Geometry check sheet. Reference: the model listing, model coordinates, mm. Face numbers are marked on the shaded views. Give positions to 0.01 mm unless a question says otherwise; leave off trailing zeros. Write each loop counter-clockwise with the first axis right and the second up, starting at its lowest first coordinate (ties: lowest second). Pieces come first, ordered by that corner, then holes. Notation, with made-up numbers: (-30.75, 85) -> (-17.75, 85) arc R28 ccw to (-17.75, 119) -> close; hole circle Ø9 at (7.25, 69). An arc over 180 degrees is marked (long way). One line per item, written item: value.
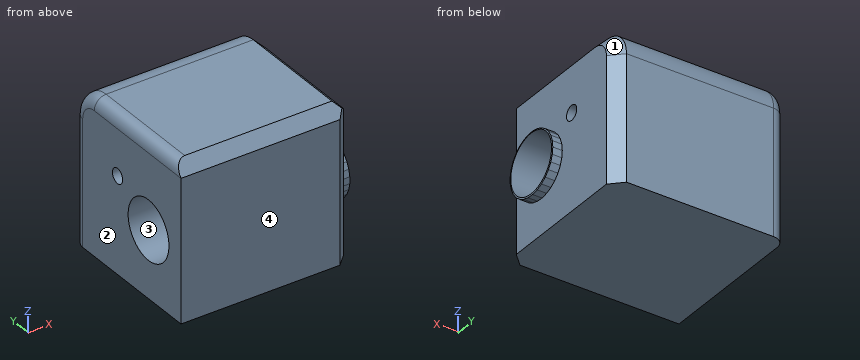
from build123d import *

# Parameters (mm, degrees)
F0_W      = 73.2621699572
F0_H      = 66.2733446807
F1_DEPTH  = 66.04
F2_R      = 12.2642048969
F4_D      = 6.35
F5_SIZE   = 5.08
F6_SIZE   = 5.08
F7_SIZE   = 5.08
F8_R      = 5.08
F10_DEPTH = 4.064
F12_D     = 25.4


with BuildPart() as f1:
    # F0 (on Top) → F1 (new body)
    with BuildSketch(Plane.XY):
        with Locations((2.2894442081, 5.3018676117)):
            Rectangle(F0_W, F0_H)
    extrude(amount=F1_DEPTH)

    # F2
    f2_edges = [f1.edges().sort_by_distance(p)[0] for p in [
        (2.289444, 38.43854, 66.04),
    ]]
    fillet(f2_edges, radius=F2_R)

    # F4 (through all)
    with Locations(Plane(origin=(-34.3416407704, 0, 0), x_dir=(0, -1, 0), z_dir=(-1, 0, 0))):
        with Locations((-11.6805844009, 41.2179939449)):
            Hole(F4_D / 2)

    # F5
    f5_edges = [f1.edges().sort_by_distance(p)[0] for p in [
        (2.289444, -27.834805, 66.04),
    ]]
    chamfer(f5_edges, length=F5_SIZE)

    # F6
    f6_edges = [f1.edges().sort_by_distance(p)[0] for p in [
        (38.920529, -27.834805, 30.48),
    ]]
    chamfer(f6_edges, length=F6_SIZE)

    # F7
    f7_edges = [f1.edges().sort_by_distance(p)[0] for p in [
        (38.920529, 34.846438, 62.447898),
    ]]
    chamfer(f7_edges, length=F7_SIZE)

    # F8
    f8_edges = [f1.edges().sort_by_distance(p)[0] for p in [
        (-34.341641, 34.846438, 62.447898),
    ]]
    fillet(f8_edges, radius=F8_R)

    # F9 (on face) → F10 (join)
    with BuildSketch(Plane.YZ.offset(38.9205291867)):
        Polygon((-1.1907316289, 16.7186320739), (1.1907316289, 18.3312571628), (3.169850874, 20.4181241781), (4.6540846899, 22.8816535376), (5.5740319532, 25.6066533465), (5.8866769522, 28.4657056424), (5.5774007542, 31.3251243174), (4.6606647705, 34.0512061324), (3.1793345569, 36.5164825315), (1.2026754677, 38.6056799302), (-1.1768861149, 40.2211097802), (-3.848084536, 41.2872363771), (-6.6860175264, 41.7542088262), (-9.5579864934, 41.6001920146), (-12.3297013601, 40.8323875974), (-14.87155982, 39.4866972558), (-17.0647073965, 37.6260439744), (-18.8065949465, 35.3374298329), (-20.015773744, 32.7278678847), (-20.6357039325, 29.9193783463), (-20.6373982652, 27.0432830671), (-20.0207775172, 24.2340650658), (-18.8146741891, 21.623080254), (-17.0754843323, 19.3324153794), (-14.8845305313, 17.4691793858), (-12.3442593509, 16.1204951174), (-9.5734510482, 15.3494255516), (-6.7016655399, 15.1920250443), (-3.8631843245, 15.6556534684), align=None)
    extrude(amount=F10_DEPTH)

    # F12 (through all)
    with Locations(Plane.YZ.offset(42.9845291867)):
        with Locations((-7.5925402343, 28.6855231971)):
            Hole(F12_D / 2)


solid = f1.part
1) Depth check by flat-ended pin: pin 1 Ø1 at (x, y) = (30, -2) entering from -Z; pin 2 Ø8 at (y, z) = (-7, 10.5) entering from +X. Enter the tip coordinate at first touch or a pass-through.
Verdict:
pin 1: z = 0
pin 2: x = 38.92
2) Sectioned sample at A-A on x = 32. Record the cut outline in (y, z) (3 decimals).
Verdict:
outline: (-27.835, 0) -> (38.439, 0) -> (38.439, 53.776) arc R12.264 ccw to (26.174, 66.04) -> (-22.755, 66.04) -> (-27.835, 60.96) -> close; hole circle Ø25.4 at (-7.593, 28.686); hole circle Ø6.35 at (11.681, 41.218)
3) Mould release check, pull along Y, two halves, no side actions. Record for the marked faces 1, 2, 3 and 4: released by +Y, released by -Y, zero draft, split by the parting line, or undercut.
Verdict:
face 1: released by +Y
face 2: zero draft
face 3: undercut
face 4: released by -Y
4) Sectioned sample at B-B on z = 4.5. Record the cut outline in (x, y), plus the area to 3 significant figures.
Verdict:
outline: (-34.34, -27.83) -> (33.84, -27.83) -> (38.92, -22.75) -> (38.92, 33.36) -> (33.84, 38.44) -> (-29.26, 38.44) arc R5.08 ccw to (-34.34, 33.36) -> close
area: 4,820 mm^2
5) Scan lines: probe 1 along X at (y, z) = (14, 54); probe 2 along Z at (x, y) = (6.5, 0.5); probe 3 along Z at (x, y) = (18, 1.5). Record each from-to range of solid material in increasing order.
Verdict:
probe 1: -34.34 to 38.92
probe 2: 0 to 18.9, 38.47 to 66.04
probe 3: 0 to 19.82, 37.55 to 66.04
6) Sectioned sample at C-C on y = 13.5. Record the cut outline in (x, z).
Verdict:
outline: (-34.34, 0) -> (38.92, 0) -> (38.92, 38.62) -> (-34.34, 38.62) -> close; (-34.34, 43.82) -> (38.92, 43.82) -> (38.92, 60.96) -> (33.84, 66.04) -> (-29.26, 66.04) arc R5.08 ccw to (-34.34, 60.96) -> close
7) Sectioned sample at D-D on y = 23.5. Record the cut outline in (x, z), plus the area to 3 significant figures.
Verdict:
outline: (-34.34, 0) -> (38.92, 0) -> (38.92, 60.96) -> (33.84, 66.04) -> (-29.26, 66.04) arc R5.08 ccw to (-34.34, 60.96) -> close
area: 4,820 mm^2
